Build history of the part. All positions in model axes, mm. A direction names the side the tool comes from. Round coordinates to 2 decimals unless told otherwise and drop trailing zeros. Write each loop counter-clockwise with the first axis right and the second up, starting at its lowest first coordinate (ties: lowest second). Pieces come first, ordered by that corner, then holes.
Item 1: Drop flat-ended pins along their axis: pin 1 Ø1 at (y, z) = (1, -5) entering from -X; pin 2 Ø1.5 at (y, z) = (1.5, -3) entering from +X. Give the stop position or say it passes through.
Item 2: Band-saw the part on B-B, the plane y = 1.3. Count the separate pieces of the cut face and the enclosed holes in it, then the cut area to 3 significant figures.
Item 3: Band-saw the part on D-D, the plane x = 29. Write the cut outline in (y, z) (1 decimal).
Item 4: Mould opens along X. For faces 1 (the cylindrical face through (-35.93, 1.61, 7.23)), 2 (the flat face through (0, 2, 9.525)), 3 (the cylindrical face through (20.27, 1.61, 0.93)) say: +X half, -X half, draft (parallel to the pull), parting line (faces both ways), or undercut.
Item 5: Band-saw the part on A-A, the plane z = -6.5. Write the cut outline in (x, y) (3 decimals), then the cut area to 3 significant figures.
Item 6: Band-saw the part on C-C, the plane x = -24.5. Write the cut outline in (y, z) (3 decimals).
Item 7: 3-axis set-ups, long thin cutter, end or side, ignore diameter. For faces 4 (the cylindrical face through (-35.93, 1.61, -7.23)), 5 (the cylindrical face through (19.611, 1.61, 4.036)): which of +Z, -Z, +X, -X, +Y, -Y reach the whole face in a straight line?
Item 8: Wall check: probe 1 along X at (y, z) = (1.3, -5.75); probe 2 along Z at (x, y) = (22, 2.9) (3 decimals); probe 3 along X at (y, z) = (1.4, 0.75). Give the ranges that are in metal, low to high.
```python
from build123d import *

# Parameters (mm, degrees)
SKETCH1_W           = 76.2
SKETCH1_H           = 19.05
BOSS_EXTRUDE1_DEPTH = 3.175
CUT_EXTRUDE1_DEPTH  = 40.400713826
FILLET1_R           = 7.62


with BuildPart() as part:
    # Sketch1 → Boss-Extrude1 (new body)
    with BuildSketch(Plane(origin=(0, 0, 0), x_dir=(1, 0, 0), z_dir=(0, 1, 0))):
        Rectangle(SKETCH1_W, SKETCH1_H)
    extrude(amount=BOSS_EXTRUDE1_DEPTH)

    # Sketch6 → Cut-Extrude1 (cut, through all)
    with BuildSketch(Plane(origin=(0, 3.175, 0), x_dir=(1, 0, 0), z_dir=(0, 1, 0))):
        with BuildLine():
            ThreePointArc((-20.158139463, 8.116433777), (-28.391214829, 4.751683872), (-33.113993118, -2.784922601))
            ThreePointArc((-33.113993118, -2.784922601), (-31.965241133, -4.713829384), (-30.03633435, -3.565077399))
            ThreePointArc((-30.03633435, -3.565077399), (-26.347053439, 2.322274641), (-19.915642535, 4.950707914))
            ThreePointArc((-19.915642535, 4.950707914), (-18.454028067, 6.654819309), (-20.158139463, 8.116433777))
        make_face()
        with BuildLine():
            ThreePointArc((-16.980295432, -1.193621711), (-20.312174356, -0.939008413), (-23.187529976, -2.641528649))
            ThreePointArc((-23.187529976, -2.641528649), (-23.064941797, -4.883243314), (-20.823227132, -4.760655135))
            ThreePointArc((-20.823227132, -4.760655135), (-19.590931867, -4.031003605), (-18.162983757, -4.14012359))
            ThreePointArc((-18.162983757, -4.14012359), (-16.098388655, -3.258216813), (-16.980295432, -1.193621711))
        make_face()
        with BuildLine():
            ThreePointArc((16.980295432, -1.193621711), (20.312174356, -0.939008413), (23.187529976, -2.641528649))
            ThreePointArc((23.187529976, -2.641528649), (23.064941797, -4.883243314), (20.823227132, -4.760655135))
            ThreePointArc((20.823227132, -4.760655135), (19.590931867, -4.031003605), (18.162983757, -4.14012359))
            ThreePointArc((18.162983757, -4.14012359), (16.098388655, -3.258216813), (16.980295432, -1.193621711))
        make_face()
        with BuildLine():
            ThreePointArc((20.158139463, 8.116433777), (28.391214829, 4.751683872), (33.113993118, -2.784922601))
            ThreePointArc((33.113993118, -2.784922601), (31.965241133, -4.713829384), (30.03633435, -3.565077399))
            ThreePointArc((30.03633435, -3.565077399), (26.347053439, 2.322274641), (19.915642535, 4.950707914))
            ThreePointArc((19.915642535, 4.950707914), (18.454028067, 6.654819309), (20.158139463, 8.116433777))
        make_face()
    extrude(amount=-CUT_EXTRUDE1_DEPTH, mode=Mode.SUBTRACT)

    # Fillet1
    fillet1_edges = [part.edges().sort_by_distance(p)[0] for p in [
        (38.1, 1.5875, 9.525),
        (-38.1, 1.5875, 9.525),
        (-38.1, 1.5875, -9.525),
        (38.1, 1.5875, -9.525),
    ]]
    fillet(fillet1_edges, radius=FILLET1_R)


solid = part.part
```
Results:
1. pin 1: stops at x = -37.64
1. pin 2: stops at x = 38.09
2. separate pieces: 1
2. enclosed holes: 4
2. area: 1,240 mm2
3. outline: (0, -9.5) - (3.2, -9.5) - (3.2, -4.2) - (0, -4.2) - close; (0, 0.9) - (3.2, 0.9) - (3.2, 9.5) - (0, 9.5) - close
4. face 1: -X half
4. face 2: draft
4. face 3: undercut
5. outline: (-36.559, 0) - (-25.787, 0) - (-25.787, 3.175) - (-36.559, 3.175) - close; (-18.45, 0) - (18.45, 0) - (18.45, 3.175) - (-18.45, 3.175) - close; (25.787, 0) - (36.559, 0) - (36.559, 3.175) - (25.787, 3.175) - close
5. area: 186 mm2
6. outline: (0, -9.525) - (3.175, -9.525) - (3.175, -7.096) - (0, -7.096) - close; (0, -3.587) - (3.175, -3.587) - (3.175, 9.525) - (0, 9.525) - close
7. face 4: -Z, -X, +Y, -Y
7. face 5: +Y, -Y
8. probe 1: x = -37.06 to -27.06, -18.66 to 18.66, 27.06 to 37.06
8. probe 2: z = -9.525 to -7.856, -4.593 to 1.642, 5.289 to 9.525
8. probe 3: x = -38.1 to -32.43, -28.9 to 28.9, 32.43 to 38.1
